Could you check a few things on this model? Use its own coordinates, in mm. Coordinates: 2 decimals unless noted, no trailing zeros.
1) Thinking about a two-plate mould opening in X: for faces 1 (the face through (0, 16, 148)), 2 (the face through (20, 4, 148)), 3 (the face through (11.48, 12.32, 147.9)), 4 (the face through (4, 20, 148)), which applies, released by +X, released by -X, zero draft, split by the parting line, or undercut?
2) Will these pins go through, and if not, where does the flat tip stop? P1, Ø1, axis at x = 0.5, z = 172.5, coming from the -Y side; P2, Ø0.7, axis at y = 19, z = 148.5, coming from the -X side; P3, Ø1, axis at x = 0.5, z = 99, coming from the +Y side.
3) If I drill on line 1 along Y through (x, z) = (2.75, 251.5); line 2 along Y through (x, z) = (10, 176), over which ranges is the centre line in solid material (lowest first)?
```python
from build123d import *

# Parameters (mm, degrees)
MODEL_R             = 2.75
BOSS_EXTRUDE1_DEPTH = 300


with BuildPart() as part:
    # Model → Boss-Extrude1 (new body)
    with BuildSketch(Plane.XY):
        with BuildLine():
            Line((1.499999935, 19.99999323), (6.799999935, 19.99999323))
            Line((6.799999935, 19.99999323), (6.799999935, 18.69999323))
            Line((6.799999935, 18.69999323), (3.999999935, 18.69999323))
            Line((3.999999935, 18.69999323), (3.999999935, 17.19999323))
            Line((3.999999935, 17.19999323), (6.745762647, 14.5))
            Line((6.745762647, 14.5), (9.565216879, 14.5))
            Line((9.565216879, 14.5), (10, 14.25))
            Line((10, 14.25), (10.434782606, 14.5))
            Line((10.434782606, 14.5), (13.254244108, 14.5))
            Line((13.254244108, 14.5), (15.999999935, 17.19999323))
            Line((15.999999935, 17.19999323), (15.999999935, 18.69999323))
            Line((15.999999935, 18.69999323), (13.199999935, 18.69999323))
            Line((13.199999935, 18.69999323), (13.199999935, 19.99999323))
            Line((13.199999935, 19.99999323), (18.499999935, 19.99999323))
            ThreePointArc((18.499999935, 19.99999323), (19.560660107, 19.560653402), (19.999999935, 18.49999323))
            Line((19.999999935, 18.49999323), (19.999999935, 13.19999323))
            Line((19.999999935, 13.19999323), (18.699999935, 13.19999323))
            Line((18.699999935, 13.19999323), (18.699999935, 15.99999323))
            Line((18.699999935, 15.99999323), (17.199999935, 15.99999323))
            Line((17.199999935, 15.99999323), (14.500000065, 13.254230518))
            Line((14.500000065, 13.254230518), (14.500000065, 10.434776138))
            Line((14.500000065, 10.434776138), (14.250000065, 9.99999323))
            Line((14.250000065, 9.99999323), (14.500000065, 9.565210911))
            Line((14.500000065, 9.565210911), (14.500000065, 6.745755942))
            Line((14.500000065, 6.745755942), (17.199999935, 3.99999323))
            Line((17.199999935, 3.99999323), (18.699999935, 3.99999323))
            Line((18.699999935, 3.99999323), (18.699999935, 6.79999323))
            Line((18.699999935, 6.79999323), (19.999999935, 6.79999323))
            Line((19.999999935, 6.79999323), (19.999999935, 1.49999323))
            ThreePointArc((19.999999935, 1.49999323), (19.560660107, 0.439333058), (18.499999935, -6.77e-06))
            Line((18.499999935, -6.77e-06), (13.199999935, -6.77e-06))
            Line((13.199999935, -6.77e-06), (13.199999935, 1.29999323))
            Line((13.199999935, 1.29999323), (15.999999935, 1.29999323))
            Line((15.999999935, 1.29999323), (15.999999935, 2.798703306))
            Line((15.999999935, 2.798703306), (13.254126104, 5.49999323))
            Line((13.254126104, 5.49999323), (10.434782606, 5.49999323))
            Line((10.434782606, 5.49999323), (10, 5.74999323))
            Line((10, 5.74999323), (9.565216879, 5.49999323))
            Line((9.565216879, 5.49999323), (6.745762647, 5.49999323))
            Line((6.745762647, 5.49999323), (3.999999935, 2.79999323))
            Line((3.999999935, 2.79999323), (3.999999935, 1.29999323))
            Line((3.999999935, 1.29999323), (6.799999935, 1.29999323))
            Line((6.799999935, 1.29999323), (6.799999935, -6.77e-06))
            Line((6.799999935, -6.77e-06), (1.499999935, -6.77e-06))
            ThreePointArc((1.499999935, -6.77e-06), (0.439339764, 0.439333058), (-6.5e-08, 1.49999323))
            Line((-6.5e-08, 1.49999323), (-6.5e-08, 6.79999323))
            Line((-6.5e-08, 6.79999323), (1.299999935, 6.79999323))
            Line((1.299999935, 6.79999323), (1.299999935, 3.99999323))
            Line((1.299999935, 3.99999323), (2.799999935, 3.99999323))
            Line((2.799999935, 3.99999323), (5.499999935, 6.745755942))
            Line((5.499999935, 6.745755942), (5.499999935, 9.565210911))
            Line((5.499999935, 9.565210911), (5.749999935, 9.99999323))
            Line((5.749999935, 9.99999323), (5.499999935, 10.434776138))
            Line((5.499999935, 10.434776138), (5.499999935, 13.254230518))
            Line((5.499999935, 13.254230518), (2.799999935, 15.99999323))
            Line((2.799999935, 15.99999323), (1.299999935, 15.99999323))
            Line((1.299999935, 15.99999323), (1.299999935, 13.19999323))
            Line((1.299999935, 13.19999323), (-6.5e-08, 13.19999323))
            Line((-6.5e-08, 13.19999323), (-6.5e-08, 18.49999323))
            ThreePointArc((-6.5e-08, 18.49999323), (0.439339764, 19.560653402), (1.499999935, 19.99999323))
        make_face()
        with Locations((10, 10)):
            Circle(MODEL_R, mode=Mode.SUBTRACT)
    extrude(amount=BOSS_EXTRUDE1_DEPTH)


solid = part.part
```
Filled in:
1. face 1: released by -X
1. face 2: released by +X
1. face 3: undercut
1. face 4: zero draft
2. P1: stops at y = 0.09
2. P2: stops at x = 0.01
2. P3: stops at y = 19.91
3. line 1: y = 0 to 4, 16 to 20
3. line 2: y = 5.75 to 7.25, 12.75 to 14.25
